For this review, take the finished solid that the model builds, in its own axes (mm). Face numbers are marked on the shaded views. A direction names the side the tool comes from. Coordinates: 2 decimals unless noted, no trailing zeros. Write each loop counter-clockwise with the first axis right and the second up, starting at its lowest first coordinate (ties: lowest second). Pieces come first, ordered by that corner, then holes. Notation, with made-up numbers: M -3,0 L 10,0 A9 cw 10,5 Z; hole C 59.5,30 d5. An arc over 180 degrees is marked long. Return JSON: item names as keys, results as strings.
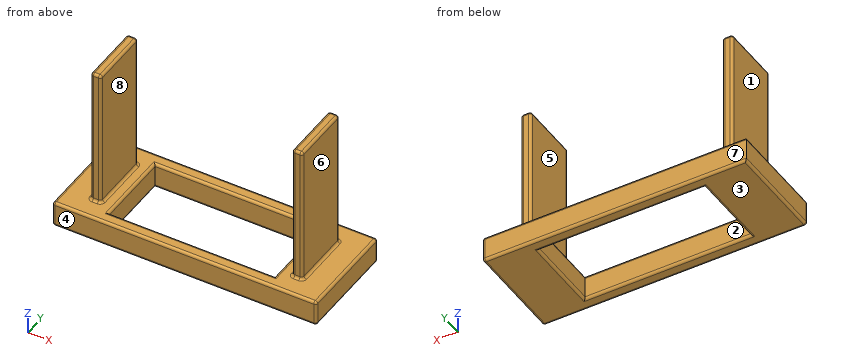
```python
from build123d import *

# Parameters (mm, degrees)
F0_W     = 103.5
F0_H     = 40
F0_W_2   = 4
F0_H_2   = 24
F1_DEPTH = 10
F2_DEPTH = 65
F3_DEPTH = 65
F4_R     = 1


with BuildPart() as f1:
    # F0 (on Top) → F1 (new body)
    with BuildSketch(Plane.XY):
        Rectangle(F0_W, F0_H)
        Polygon((-37.5, 12), (-37.5, 0), (-37.5, -12), (-41.5, -12), (-41.5, 12), align=None, mode=Mode.SUBTRACT)
        Polygon((32.5, -15), (-32.5, -15), (-32.5, 0), (-32.5, 15), (32.5, 15), align=None, mode=Mode.SUBTRACT)
        with Locations((39.5, 0)):
            Rectangle(F0_W_2, F0_H_2, mode=Mode.SUBTRACT)
    extrude(amount=F1_DEPTH)

    # F0 (on Top) → F2 (join)
    with BuildSketch(Plane.XY):
        Polygon((-37.5, -12), (-37.5, 0), (-37.5, 12), (-41.5, 12), (-41.5, -12), align=None)
    extrude(amount=F2_DEPTH)

    # F0 (on Top) → F3 (join)
    with BuildSketch(Plane.XY):
        with Locations((39.5, 0)):
            Rectangle(F0_W_2, F0_H_2)
    extrude(amount=F3_DEPTH)

    # F4
    f4_edges = [f1.edges().sort_by_distance(p)[0] for p in [
        (-51.75, -20, 5),
        (51.75, -20, 5),
        (0, -20, 0),
        (0, -20, 10),
        (51.75, 20, 5),
        (51.75, 0, 0),
        (51.75, 0, 10),
        (0, 20, 10),
        (-51.75, 0, 10),
        (-37.5, 0, 10),
        (-39.5, -12, 10),
        (-41.5, 0, 10),
        (-39.5, 12, 10),
        (0, -15, 10),
        (-32.5, 0, 10),
        (0, 15, 10),
        (32.5, 0, 10),
        (39.5, 12, 10),
        (41.5, 0, 10),
        (39.5, -12, 10),
        (37.5, 0, 10),
        (37.5, 12, 37.5),
        (39.5, 12, 65),
        (41.5, 12, 37.5),
        (41.5, 0, 65),
        (37.5, 0, 65),
        (39.5, -12, 65),
        (-41.5, 12, 37.5),
        (-39.5, 12, 65),
        (-37.5, 12, 37.5),
        (41.5, -12, 37.5),
        (37.5, -12, 37.5),
        (-37.5, 0, 65),
        (-37.5, -12, 37.5),
        (-39.5, -12, 65),
        (-41.5, -12, 37.5),
        (-41.5, 0, 65),
        (0, 20, 0),
        (-51.75, 0, 0),
        (0, -15, 0),
        (-32.5, 0, 0),
        (0, 15, 0),
        (32.5, 0, 0),
    ]]
    fillet(f4_edges, radius=F4_R)


solid = f1.part
```
1. We need section C-C (z = 48.5). State the section outline as (x, y) points, plus the area to 3 significant figures.
Checks:
{"outline": "M -41.5,-11 A1 ccw -40.5,-12 L -38.5,-12 A1 ccw -37.5,-11 L -37.5,11 A1 ccw -38.5,12 L -40.5,12 A1 ccw -41.5,11 Z; M 37.5,-11 A1 ccw 38.5,-12 L 40.5,-12 A1 ccw 41.5,-11 L 41.5,11 A1 ccw 40.5,12 L 38.5,12 A1 ccw 37.5,11 Z", "area": "190 mm2"}
2. We need section B-B (x = -1). State the section outline as (y, z) points.
Checks:
{"outline": "M -20,1 A1 ccw -19,0 L -16,0 A1 ccw -15,1 L -15,9 A1 ccw -16,10 L -19,10 A1 ccw -20,9 Z; M 15,1 A1 ccw 16,0 L 19,0 A1 ccw 20,1 L 20,9 A1 ccw 19,10 L 16,10 A1 ccw 15,9 Z"}
3. Clearance check with flat-ended pins moving along their axes: pin 1 Ø1.6 at (x, z) = (39, 27.5) entering from -Y; pin 2 Ø6.5 at (y, z) = (2.5, 42.5) entering from +X; pin 3 Ø17.5 at (y, z) = (3.5, 32) entering from -X. State where each tip first meets the part, or that it passes through.
Checks:
{"pin 1": "y = -12", "pin 2": "x = 41.5", "pin 3": "x = -41.5"}
4. Wall thickness on L1, parallel to X at y = 4.5, z = 49.5; L2, parallel to Y at x = -24, z = 7; L3, parallel to X at y = -9.5, z = 4: over which ranges is each line inside the solid? List them lowest first. Write a range as from..to.
Checks:
{"L1": "-41.5..-37.5, 37.5..41.5", "L2": "-20..-15, 15..20", "L3": "-51.75..-32.5, 32.5..51.75"}
5. Draft analysis for pull direction X (two halves, no side actions). For the marked faces 6, 7 and 8, state which applies: +X half, -X half, draft (parallel to the pull), parting line (faces both ways), or undercut.
Checks:
{"face 6": "+X half", "face 7": "draft", "face 8": "undercut"}
6. For the marked faces 1, 2, 3, 4 and 5, list the 3-axis set-ups (+Z, -Z, +X, -X, +Y, -Y) from which the entire face can be reached by the end or side of a thin tool; tool diameter is ignored.
Checks:
{"face 1": "+Z, -X, +Y, -Y", "face 2": "+Z, -Z", "face 3": "-Z, +X, -X, +Y, -Y", "face 4": "+Z, -Z, +X, -X, -Y", "face 5": "+Z, +Y, -Y"}
